The drawing under review shows one solid part. Ordinate dimensions are in mm from its lowest x, y, z. A direction names the side the tool comes from. Coordinates: 2 decimals unless noted, no trailing zeros. Write each loop counter-clockwise with the first axis right and the second up, starting at its lowest first coordinate (ties: lowest second). Pieces come first, ordered by that corner, then holes. Notation, with made-up numbers: (16, 44.25) -> (45, 44.25) arc R18 cw to (45, 78.25) -> close; hole circle Ø6 at (37, 34.5). An arc over 180 degrees is marked (long way). One line per question, with ' | ' between items. Start each with the question number.
Q1. For P1, Ø2, axis at x = 17, y = 21.5, coming from the -Z side; P2, Ø1.5, axis at y = 18.5, z = 27.5, coming from the -X side; P3, Ø12, axis at y = 30, z = 35, coming from the +X side; P4, Ø12, axis at y = 44, z = 46, coming from the +X side, all flat-tipped, find the tip position at first contact; note any pin that passes through.
Q2. Add section C-C on z = 31. State the section outline as (x, y) points.
Q3. Draft analysis for pull direction Y (two halves, no side actions). For the marked faces 1, 2 and 3, state which applies: pulls with the +Y half, pulls with the -Y half, needs draft (parallel to the pull), parting line crosses it, or undercut.
Q4. For the marked faces 4, 5 and 6, list the 3-axis set-ups (+Z, -Z, +X, -X, +Y, -Y) from which the entire face can be reached by the end or side of a thin tool; tool diameter is ignored.
Q5. Add section B-B on y = 27. State the section outline as (x, z) points.
Q6. Add section A-A on x = 25. State the section outline as (y, z) points, and give its area (3 significant figures).
Q7. Add section D-D on z = 21.5. State the section outline as (x, y) points.
Q8. Wall thickness on probe 1 along X at (y, z) = (36, 51); probe 2 along Y at (x, z) = (25, 16); probe 3 along X at (y, z) = (5.5, 3): over which ranges is each line inside the solid? List them lowest first.
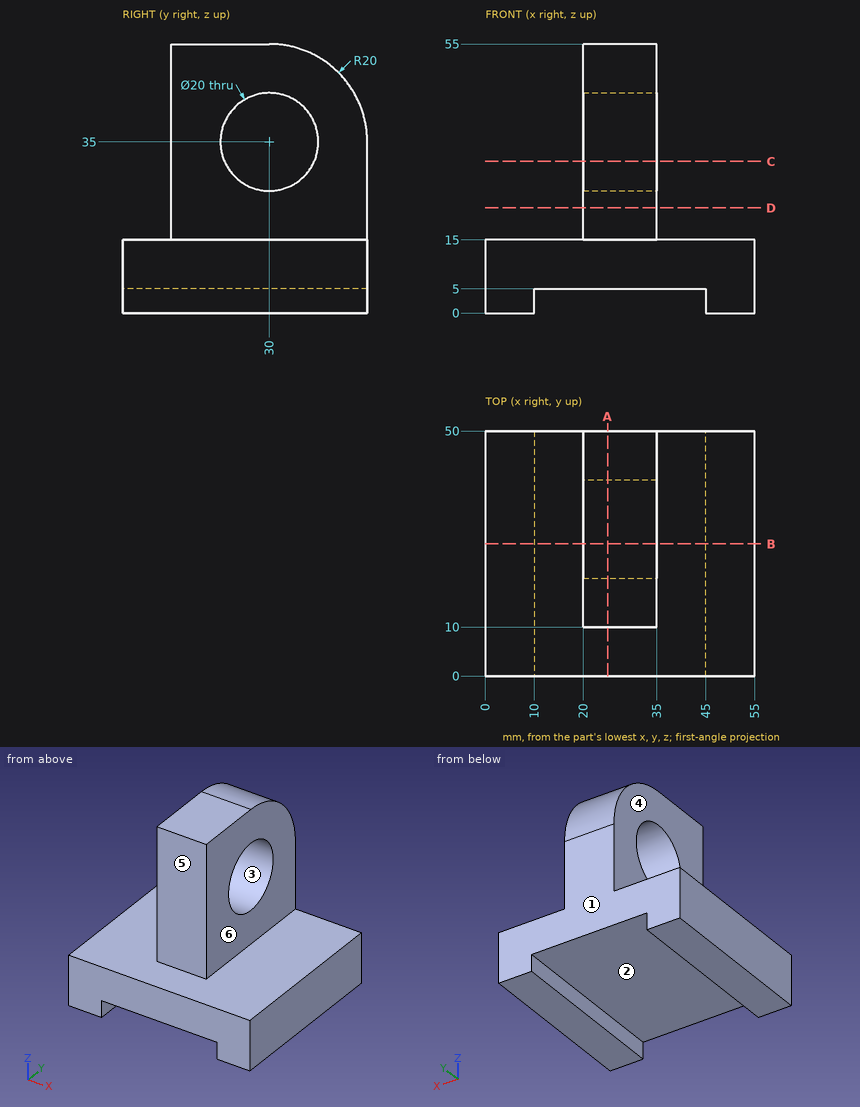
Output values:
1) P1: stops at z = 5 | P2: stops at x = 20 | P3: passes through | P4: stops at x = 35
2) outline: (20, 10) -> (35, 10) -> (35, 20.83) -> (20, 20.83) -> close; (20, 39.17) -> (35, 39.17) -> (35, 50) -> (20, 50) -> close
3) face 1: pulls with the +Y half | face 2: needs draft | face 3: undercut
4) face 4: +Z, -X, +Y, -Y | face 5: +Z, +X, -X, -Y | face 6: +Z, +X, +Y, -Y
5) outline: (0, 0) -> (10, 0) -> (10, 5) -> (45, 5) -> (45, 0) -> (55, 0) -> (55, 15) -> (35, 15) -> (35, 25.46) -> (20, 25.46) -> (20, 15) -> (0, 15) -> close; (20, 44.54) -> (35, 44.54) -> (35, 55) -> (20, 55) -> close
6) outline: (0, 5) -> (50, 5) -> (50, 35) arc R20 ccw to (30, 55) -> (10, 55) -> (10, 15) -> (0, 15) -> close; hole circle Ø20 at (30, 35) | area: 1,700 mm2
7) outline: (20, 10) -> (35, 10) -> (35, 50) -> (20, 50) -> close
8) probe 1: x = 20 to 35 | probe 2: y = 10 to 50 | probe 3: x = 0 to 10, 45 to 55
